For this review, take the finished solid that the model builds, in its own axes (mm). A direction names the side the tool comes from. Coordinates: 2 decimals unless noted, no trailing zeros. Write each loop counter-clockwise with the first axis right and the second up, starting at its lowest first coordinate (ties: lowest second). Pieces come first, ordered by that corner, then holes. Notation, with made-up numbers: (60.5, 45) -> (87.5, 45) arc R34 cw to (87.5, 83) -> close; hole circle Ø9 at (-21, 8). An arc over 180 degrees is marked (long way). One line per item, written item: value. Start each with the question number.
1) Add section A-A (z = 0). State the section outline as (x, y) points.
2) For pin 1 Ø8 at (x, z) = (12, 16) entering from +Y; pin 2 Ø2.5 at (x, y) = (13, -66) entering from -Z; pin 3 Ø4.5 at (x, y) = (25.5, 0.5) entering from +Z; pin 4 Ø1.2 at (x, y) = (26, 60.5) entering from +Z, all flat-tipped, find the tip position at first contact; note any pin that passes through.
3) Machinability: for faces 3 (the flat face through (26, 0, 66)), 4 (the cylindrical face through (13.804, 64.945, -2.668)), which of the approach directions +Z, -Z, +X, -X, +Y, -Y give a long, thin tool a straight path to every point of the face, cutting with its end or side? Answer none if there is none.
4) Mouldability with a two-part tool opening along Z and no side actions: class faces 1 (the flat face through (26.03, -57.14, -33.03)), 2 (the cylindrical face through (13.804, 74.362, 9.764)) as released by +Z, released by -Z, zero draft, split by the parting line, or undercut.
5) For probe 1 along Y at (x, z) = (15.5, -35); probe 2 along Y at (x, z) = (24, -55.5); probe 3 along Z at (x, y) = (2.25, -46.5), list the stretches that pass through material, from the lowest coordinate up. Write a range as from..to.
6) Add section B-B (y = 50). State the section outline as (x, z) points.
7) Add section C-C (x = 3). State the section outline as (y, z) points, and give its area (3 significant figures).
8) Add section D-D (x = 26). State how many separate pieces and enclosed holes the cut face has, and give its area (3 significant figures).
from build123d import *

# Parameters (mm, degrees)
SKETCH1_R           = 75
SKETCH1_R_2         = 65
BOSS_EXTRUDE1_DEPTH = 28
CUT_EXTRUDE1_REACH  = 111.7
CUT_EXTRUDE2_REACH  = 111.7
SKETCH3_R           = 2.65
CUT_EXTRUDE3_DEPTH  = 4


with BuildPart() as part:
    # Sketch1 → Boss-Extrude1 (new body)
    with BuildSketch(Plane(origin=(0, 0, 0), x_dir=(0, 0, -1), z_dir=(1, 0, 0))):
        Circle(SKETCH1_R)
        Circle(SKETCH1_R_2, mode=Mode.SUBTRACT)
    extrude(amount=BOSS_EXTRUDE1_DEPTH)

    # Sketch2 → Cut-Extrude1 (cut, up to next)
    with BuildSketch(Plane(origin=(28, 0, 0), x_dir=(0, 0, -1), z_dir=(1, 0, 0)), mode=Mode.PRIVATE) as cut_extrude1_sk1:
        with BuildLine():
            Line((-13.5, -51.893967527), (13.5, -51.893967527))
            Line((13.5, -51.893967527), (13.5, -69))
            ThreePointArc((13.5, -69), (13.207106781, -69.707106781), (12.5, -70))
            Line((12.5, -70), (-12.5, -70))
            ThreePointArc((-12.5, -70), (-13.207106781, -69.707106781), (-13.5, -69))
            Line((-13.5, -69), (-13.5, -51.893967527))
        make_face()
    cut_extrude1_tool1 = extrude(cut_extrude1_sk1.sketch, amount=-CUT_EXTRUDE1_REACH, mode=Mode.PRIVATE) & part.part
    add(cut_extrude1_tool1.solids().sort_by_distance((28, -60.939225, 0))[0], mode=Mode.SUBTRACT)

    # Sketch3 → Cut-Extrude2 (cut, up to next)
    with BuildSketch(Plane(origin=(28, 0, 0), x_dir=(0, 0, -1), z_dir=(1, 0, 0)), mode=Mode.PRIVATE) as cut_extrude2_sk1:
        with Locations((-70, 0)):
            Circle(SKETCH3_R)
    cut_extrude2_tool1 = extrude(cut_extrude2_sk1.sketch, amount=-CUT_EXTRUDE2_REACH, mode=Mode.PRIVATE) & part.part
    # Sketch3 → Cut-Extrude2 (cut, up to next)
    with BuildSketch(Plane(origin=(28, 0, 0), x_dir=(0, 0, -1), z_dir=(1, 0, 0)), mode=Mode.PRIVATE) as cut_extrude2_sk2:
        with Locations((-35, 60.621778265)):
            Circle(SKETCH3_R)
    cut_extrude2_tool2 = extrude(cut_extrude2_sk2.sketch, amount=-CUT_EXTRUDE2_REACH, mode=Mode.PRIVATE) & part.part
    # Sketch3 → Cut-Extrude2 (cut, up to next)
    with BuildSketch(Plane(origin=(28, 0, 0), x_dir=(0, 0, -1), z_dir=(1, 0, 0)), mode=Mode.PRIVATE) as cut_extrude2_sk3:
        with Locations((35, 60.621778265)):
            Circle(SKETCH3_R)
    cut_extrude2_tool3 = extrude(cut_extrude2_sk3.sketch, amount=-CUT_EXTRUDE2_REACH, mode=Mode.PRIVATE) & part.part
    # Sketch3 → Cut-Extrude2 (cut, up to next)
    with BuildSketch(Plane(origin=(28, 0, 0), x_dir=(0, 0, -1), z_dir=(1, 0, 0)), mode=Mode.PRIVATE) as cut_extrude2_sk4:
        with Locations((70, 0)):
            Circle(SKETCH3_R)
    cut_extrude2_tool4 = extrude(cut_extrude2_sk4.sketch, amount=-CUT_EXTRUDE2_REACH, mode=Mode.PRIVATE) & part.part
    # Sketch3 → Cut-Extrude2 (cut, up to next)
    with BuildSketch(Plane(origin=(28, 0, 0), x_dir=(0, 0, -1), z_dir=(1, 0, 0)), mode=Mode.PRIVATE) as cut_extrude2_sk5:
        with Locations((35, -60.621778265)):
            Circle(SKETCH3_R)
    cut_extrude2_tool5 = extrude(cut_extrude2_sk5.sketch, amount=-CUT_EXTRUDE2_REACH, mode=Mode.PRIVATE) & part.part
    # Sketch3 → Cut-Extrude2 (cut, up to next)
    with BuildSketch(Plane(origin=(28, 0, 0), x_dir=(0, 0, -1), z_dir=(1, 0, 0)), mode=Mode.PRIVATE) as cut_extrude2_sk6:
        with Locations((-35, -60.621778265)):
            Circle(SKETCH3_R)
    cut_extrude2_tool6 = extrude(cut_extrude2_sk6.sketch, amount=-CUT_EXTRUDE2_REACH, mode=Mode.PRIVATE) & part.part
    add(cut_extrude2_tool1.solids().sort_by_distance((28, 0, 70))[0], mode=Mode.SUBTRACT)
    add(cut_extrude2_tool2.solids().sort_by_distance((28, 60.621778, 35))[0], mode=Mode.SUBTRACT)
    add(cut_extrude2_tool3.solids().sort_by_distance((28, 60.621778, -35))[0], mode=Mode.SUBTRACT)
    add(cut_extrude2_tool4.solids().sort_by_distance((28, 0, -70))[0], mode=Mode.SUBTRACT)
    add(cut_extrude2_tool5.solids().sort_by_distance((28, -60.621778, -35))[0], mode=Mode.SUBTRACT)
    add(cut_extrude2_tool6.solids().sort_by_distance((28, -60.621778, 35))[0], mode=Mode.SUBTRACT)

    # Sketch4 → Cut-Extrude3 (cut)
    with BuildSketch(Plane(origin=(28, 0, 0), x_dir=(0, 0, -1), z_dir=(1, 0, 0))):
        Polygon((-39, 58.312377188), (-35, 56.002976111), (-31, 58.312377188), (-31, 62.931179342), (-35, 65.240580418), (-39, 62.931179342), align=None)
        Polygon((-70, -4.618802154), (-66, -2.309401077), (-66, 2.309401077), (-70, 4.618802154), (-74, 2.309401077), (-74, -2.309401077), align=None)
        Polygon((31, 62.931179342), (31, 58.312377188), (35, 56.002976111), (39, 58.312377188), (39, 62.931179342), (35, 65.240580418), align=None)
        Polygon((70, 4.618802154), (66, 2.309401077), (66, -2.309401077), (70, -4.618802154), (74, -2.309401077), (74, 2.309401077), align=None)
        Polygon((39, -58.312377188), (35, -56.002976111), (31, -58.312377188), (31, -62.931179342), (35, -65.240580418), (39, -62.931179342), align=None)
        Polygon((-31, -62.931179342), (-31, -58.312377188), (-35, -56.002976111), (-39, -58.312377188), (-39, -62.931179342), (-35, -65.240580418), align=None)
    extrude(amount=-CUT_EXTRUDE3_DEPTH, mode=Mode.SUBTRACT)


solid = part.part
Numbers:
1. outline: (0, -75) -> (28, -75) -> (28, -70) -> (0, -70) -> close; (0, 65) -> (28, 65) -> (28, 75) -> (0, 75) -> close
2. pin 1: y = 74.03
2. pin 2: z = -37.85
2. pin 3: z = 75
2. pin 4: z = 45.13
3. face 3: +X
3. face 4: +X, -X
4. face 1: undercut
4. face 2: split by the parting line
5. probe 1: -66.33..-63.27, -57.97..-54.77, 54.77..57.97, 63.27..66.33
5. probe 2: -50.45..-33.83, 33.83..50.45
5. probe 3: -58.85..-45.42, 45.42..58.85
6. outline: (0, -55.9) -> (28, -55.9) -> (28, -41.53) -> (0, -41.53) -> close; (0, 41.53) -> (28, 41.53) -> (28, 55.9) -> (0, 55.9) -> close
7. outline: circle Ø150 at (0, 0); hole (-70, -12.5) arc R1 ccw to (-69, -13.5) -> (-63.58, -13.5) arc R65 ccw (long way) to (-63.58, 13.5) -> (-69, 13.5) arc R1 ccw to (-70, 12.5) -> close; hole circle Ø5.3 at (-60.62, -35); hole circle Ø5.3 at (-60.62, 35); hole circle Ø5.3 at (0, -70); hole circle Ø5.3 at (0, 70); hole circle Ø5.3 at (60.62, -35); hole circle Ø5.3 at (60.62, 35)
7. area: 4,120 mm²
8. separate pieces: 1
8. enclosed holes: 7
8. area: 3,920 mm²
